Work out the finished part from the listing and answer in its coordinate system (mm). A direction names the side the tool comes from. Give positions to 0.01 mm unless a question says otherwise; leave off trailing zeros. Loops run counter-clockwise (first coordinate to the right, second up) from the corner with the lowest first, then second, coordinate; pieces in that order, holes last. Notation, with made-up numbers: (58.5, 86.5) - (80.5, 86.5) arc R20 ccw to (80.5, 98.5) - close; hole circle Ø3 at (3.25, 3.5). An arc over 180 degrees is marked (long way). One line per item, written item: value.
from build123d import *

# Parameters (mm, degrees)
F0_R     = 1.5
F0_R_2   = 1.25
F1_DEPTH = 10
F3_R     = 1.75
F3_R_2   = 1.5
F4_DEPTH = 3


with BuildPart() as f1:
    # F0 (on Right) → F1 (new body)
    with BuildSketch(Plane.YZ):
        Circle(F0_R)
        Circle(F0_R_2, mode=Mode.SUBTRACT)
    extrude(amount=F1_DEPTH)

    # F3 (on offset) → F4 (join)
    with BuildSketch(Plane.YZ.offset(1.71)):
        Circle(F3_R)
        Circle(F3_R_2, mode=Mode.SUBTRACT)
    extrude(amount=F4_DEPTH)


solid = f1.part
1. Flat-ended cylindrical pins translate along their axes: pin 1 Ø1 at (x, y) = (2, 1.5) entering from +Z; pin 2 Ø1.5 at (x, z) = (5.5, -1.5) entering from -Y. Find the tip coordinate at first contact, or state that the pin passes through.
Output:
pin 1: stops at z = 1.44
pin 2: stops at y = -1.3
2. The mould has two halves that part along Z. Classify faces 3 (the cylindrical face through (0.84, -1.5, 0.07)), 4 (the cylindrical face through (4.93, -0.27, -1.22)): released by +Z, released by -Z, zero draft, split by the parting line, or undercut.
Output:
face 3: split by the parting line
face 4: undercut
3. Find the intervals of material crossed by line 1 along Y through (x, z) = (7.5, 0.05); line 2 along Z through (x, y) = (4.25, 0), in increasing order.
Output:
line 1: y = -1.5 to -1.25, 1.25 to 1.5
line 2: z = -1.75 to -1.25, 1.25 to 1.75
4. Section C-C (x = 8.25) is taken. Write down the section's boundary in (y, z).
Output:
outline: circle Ø3 at (0, 0); hole circle Ø2.5 at (0, 0)
5. For faces 1 (the cylindrical face through (3.189, 1.617, -0.67)), 2 (the cylindrical face through (7.32, -1.5, 0.07)), determine the directions among +Z, -Z, +X, -X, +Y, -Y from which every point of the face is accessible in a straight line to the end or side of a thin tool.
Output:
face 1: +X, -X
face 2: +X
6. Section A-A (y = 0) is taken. Write down the section's boundary in (x, z), and give its area (3 significant figures).
Output:
outline: (0, -1.5) - (1.71, -1.5) - (1.71, -1.75) - (4.71, -1.75) - (4.71, -1.5) - (10, -1.5) - (10, -1.25) - (0, -1.25) - close; (0, 1.25) - (10, 1.25) - (10, 1.5) - (4.71, 1.5) - (4.71, 1.75) - (1.71, 1.75) - (1.71, 1.5) - (0, 1.5) - close
area: 6.50 mm²
7. Section D-D (y = 1.35) is taken. Write down the section's boundary in (x, z).
Output:
outline: (0, -0.65) - (1.71, -0.65) - (1.71, -1.11) - (4.71, -1.11) - (4.71, -0.65) - (10, -0.65) - (10, 0.65) - (4.71, 0.65) - (4.71, 1.11) - (1.71, 1.11) - (1.71, 0.65) - (0, 0.65) - close
